Geometry check sheet. Reference: the model listing, model coordinates, mm. Face numbers are marked on the shaded views. Coordinates: 2 decimals unless noted, no trailing zeros. Loops run counter-clockwise (first coordinate to the right, second up) from the corner with the lowest first, then second, coordinate; pieces in that order, holes last. Notation, with made-up numbers: (52, 21) - (63, 21) arc R27 cw to (63, 38) - close; hole circle Ø1 at (-12, -9). An arc over 180 degrees is marked (long way). Write each question's results on one line, items separated by ' | '. Start each with the question number.
(1) Go/stop test with flat-tipped pins: pin 1 Ø1.5 at (x, z) = (7.25, 0) entering from +Y; pin 2 Ø3 at (x, z) = (-7.25, 0) entering from -Y. Record where each tip stops, or that it passes through.
(2) Sectioned sample at D-D (y = 0.3). State how many separate pieces and enclosed holes the cut face has, plus the area to 3 significant figures.
(3) Sectioned sample at A-A (z = 0). Enter the section's corners in (x, y).
(4) Sectioned sample at C-C (x = -2). Enter the section's corners in (y, z).
(5) Material ranges on probe 1 along X at (y, z) = (0.9, 0); probe 2 along X at (y, z) = (1.1, 0); probe 3 along Z at (x, y) = (8, 0.45), recorded low to high.
(6) Mould release check, pull along X, two halves, no side actions. Record for the marked faces 1 and 2: pulls with the +X half, pulls with the -X half, needs draft (parallel to the pull), parting line crosses it, or undercut.
(7) Sectioned sample at B-B (x = -7.25). Enter the section's corners in (y, z), plus the area to 3 significant figures.
from build123d import *

# Parameters (mm, degrees)
SKETCH1_W                 = 18.8
SKETCH1_H                 = 14
SKETCH1_R                 = 1.25
CABLE_PLATE_EXTRUDE_DEPTH = 1.4
FILLET2_R                 = 1
FILLET1_R                 = 0.6


with BuildPart() as part:
    # Sketch1 → Cable Plate Extrude (new body)
    with BuildSketch(Plane(origin=(0, 0, 0), x_dir=(1, 0, 0), z_dir=(0, 1, 0))):
        Rectangle(SKETCH1_W, SKETCH1_H)
        with Locations(Location((-7.25, 0, 0), (0, 0, 270))):
            Circle(SKETCH1_R, mode=Mode.SUBTRACT)
        with Locations(Location((7.25, 0, 0), (0, 0, 270))):
            Circle(SKETCH1_R, mode=Mode.SUBTRACT)
    extrude(amount=CABLE_PLATE_EXTRUDE_DEPTH)

    # Fillet2
    fillet2_edges = [part.edges().sort_by_distance(p)[0] for p in [
        (-9.4, 0.7, -7),
        (9.4, 0.7, -7),
        (9.4, 0.7, 7),
        (-9.4, 0.7, 7),
    ]]
    fillet(fillet2_edges, radius=FILLET2_R)

    # Fillet1
    fillet1_edges = [part.edges().sort_by_distance(p)[0] for p in [
        (0, 0, 7),
        (0, 1.4, 7),
        (-9.4, 0, 0),
        (0, 0, -7),
        (9.4, 0, 0),
        (-9.107106781, 0, -6.707106781),
        (9.107106781, 0, -6.707106781),
        (9.107106781, 0, 6.707106781),
        (-9.107106781, 0, 6.707106781),
        (-9.4, 1.4, 0),
        (9.4, 1.4, 0),
        (0, 1.4, -7),
        (-9.107106781, 1.4, -6.707106781),
        (9.107106781, 1.4, -6.707106781),
        (9.107106781, 1.4, 6.707106781),
        (-9.107106781, 1.4, 6.707106781),
    ]]
    fillet(fillet1_edges, radius=FILLET1_R)


solid = part.part
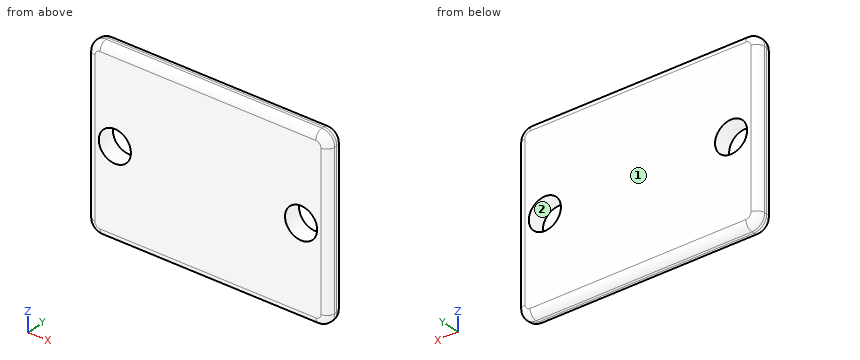
Outcome:
1) pin 1: passes through | pin 2: stops at y = 0
2) separate pieces: 1 | enclosed holes: 2 | area: 247 mm2
3) outline: (-9.4, 0.6) arc R0.6 ccw to (-8.8, 0) - (-8.5, 0) - (-8.5, 1.4) - (-8.8, 1.4) arc R0.6 ccw to (-9.4, 0.8) - close; (-6, 0) - (6, 0) - (6, 1.4) - (-6, 1.4) - close; (8.5, 0) - (8.8, 0) arc R0.6 ccw to (9.4, 0.6) - (9.4, 0.8) arc R0.6 ccw to (8.8, 1.4) - (8.5, 1.4) - close
4) outline: (0, -6.4) arc R0.6 ccw to (0.6, -7) - (0.8, -7) arc R0.6 ccw to (1.4, -6.4) - (1.4, 6.4) arc R0.6 ccw to (0.8, 7) - (0.6, 7) arc R0.6 ccw to (0, 6.4) - close
5) probe 1: x = -9.39 to -8.5, -6 to 6, 8.5 to 9.39 | probe 2: x = -9.32 to -8.5, -6 to 6, 8.5 to 9.32 | probe 3: z = -6.98 to -1, 1 to 6.98
6) face 1: needs draft | face 2: undercut
7) outline: (0, -6.4) arc R0.6 ccw to (0.6, -7) - (0.8, -7) arc R0.6 ccw to (1.4, -6.4) - (1.4, -1.25) - (0, -1.25) - close; (0, 1.25) - (1.4, 1.25) - (1.4, 6.4) arc R0.6 ccw to (0.8, 7) - (0.6, 7) arc R0.6 ccw to (0, 6.4) - close | area: 15.8 mm2
